Input: part model. Units: mm. Frame: model coordinates. Round coordinates to 2 decimals unless told otherwise and drop trailing zeros. Write each loop counter-clockwise with the first axis right and the second up, starting at its lowest first coordinate (ties: lowest second). Pieces come first, ordered by that corner, then holes. Notation, with made-up numbers: M 51.25,45.5 L 77.25,45.5 A10 ccw 77.25,55.5 Z; hole C 13.25,46.25 d7. An arc over 180 degrees is marked long. Answer as CSV lines item,"result". Start each with the question number.
```python
from build123d import *

# Parameters (mm, degrees)
SKETCH1_W           = 8.89
SKETCH1_H           = 19.05
SKETCH1_R           = 1.4605
BOSS_EXTRUDE1_DEPTH = 3.175
FILLET1_R           = 6.35


with BuildPart() as part:
    # Sketch1 → Boss-Extrude1 (new body)
    with BuildSketch(Plane(origin=(0, 0, 0), x_dir=(1, 0, 0), z_dir=(0, 1, 0))):
        with Locations((4.445, 9.525)):
            Rectangle(SKETCH1_W, SKETCH1_H)
        with Locations(Location((4.445, 15.24, 0), (0, 0, 270))):
            Circle(SKETCH1_R, mode=Mode.SUBTRACT)
    extrude(amount=BOSS_EXTRUDE1_DEPTH)

    # Fillet1
    # the kernel refuses this fillet: 6.35 mm, written as the material it takes off along each edge
    with BuildSketch(Plane(origin=(8.89, -15.875, -19.05), x_dir=(0, 0, 1), z_dir=(0, 1, 0)), Plane(origin=(0, -15.875, -19.05), x_dir=(1, 0, 0), z_dir=(0, 1, 0))) as fillet1_piece_1:
        with BuildLine():
            CenterArc((FILLET1_R, -FILLET1_R), FILLET1_R, 90, 90)
            Line((0, -FILLET1_R), (0, 0))
            Line((0, 0), (FILLET1_R, 0))
        make_face()
    extrude(amount=34.925, mode=Mode.SUBTRACT)


solid = part.part
```
Item 1: Draft query along X for faces 1 (the face through (4, 2, 0)), 2 (the face through (7.7, 1.6, -16.4)), 3 (the face through (3.89, 1.57, -13.89)). Return one class per face: +X half, -X half, draft (parallel to the pull), parting line (faces both ways), or undercut.
Item 2: Cut plane B-B, the plane x = 4.75. Return loops of the section in (y, z) (3 decimals).
Item 3: Cut plane D-D, the plane x = 2. Return loops of the section in (y, z) (3 decimals).
Item 4: Cut plane A-A, the plane z = -15.24. Return loops of the section in (x, y) (1 decimal), plus the area to 3 significant figures.
Item 5: Line query: line 1 (Z direction, x = 4.75, y = 0.6); line 2 (Z direction, x = 5.75, y = 1.6); line 3 (X direction, y = 2.25, z = -15.24). Output: solid intervals per line, ascending. Write a range as [from, to].
Results list:
1,face 1,"draft"
1,face 2,"+X half"
1,face 3,"undercut"
2,outline,"M 0,-18.653 L 3.175,-18.653 L 3.175,-16.668 L 0,-16.668 Z; M 0,-13.812 L 3.175,-13.812 L 3.175,0 L 0,0 Z"
3,outline,"M 0,-17.326 L 3.175,-17.326 L 3.175,0 L 0,0 Z"
4,outline,"M 0.5,0 L 3,0 L 3,3.2 L 0.5,3.2 Z; M 5.9,0 L 8.4,0 L 8.4,3.2 L 5.9,3.2 Z"
4,area,"15.6 mm²"
5,line 1,"[-18.65, -16.67], [-13.81, 0]"
5,line 2,"[-18.18, -15.9], [-14.58, 0]"
5,line 3,"[0.53, 2.98], [5.91, 8.36]"
